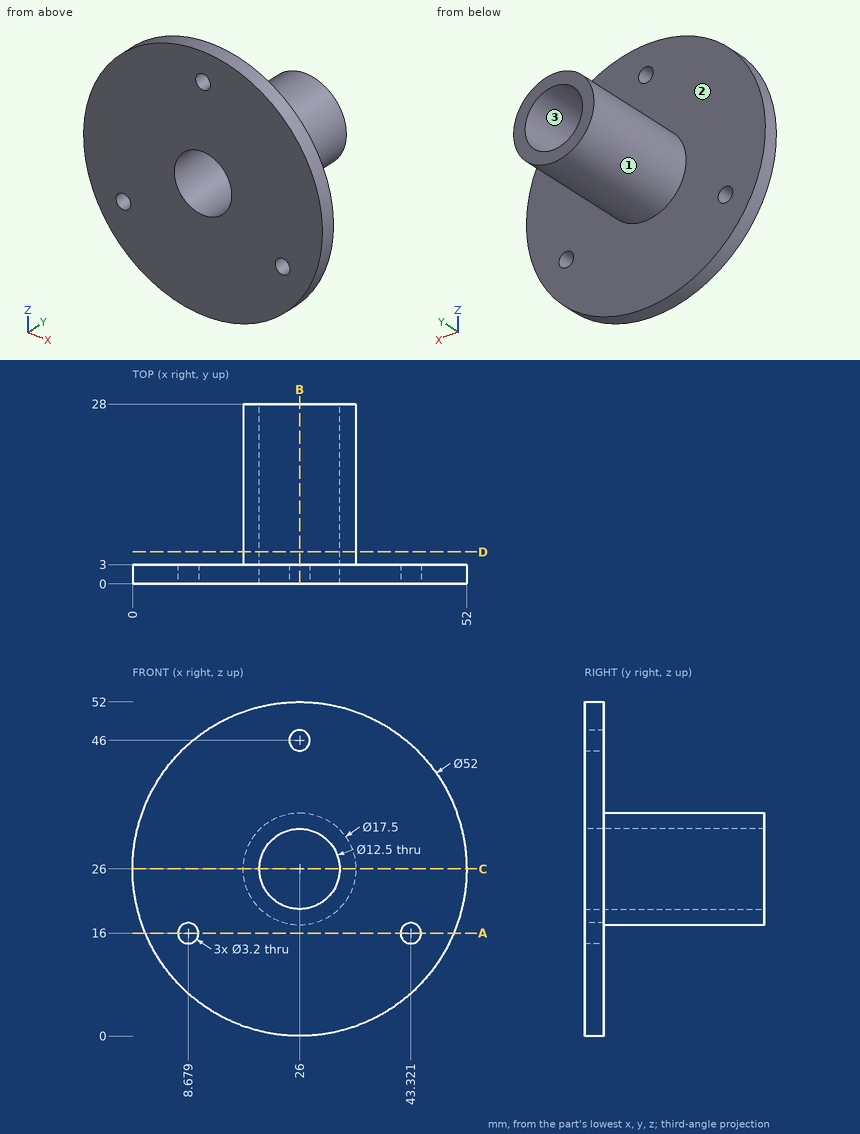
The figure shows three views and two pictorial views of one solid part (mm, origin at its lowest corner). Answer the questions. Coordinates: 2 decimals unless noted, no trailing zeros. Loops run counter-clockwise (first coordinate to the right, second up) from the corner with the lowest first, then second, coordinate; pieces in that order, holes last. Notation, with made-up numbers: M 51,69 L 72,69 A10 ccw 72,84 Z; hole C 53.25,42.25 d8. An arc over 180 degrees is marked long. Answer as CSV lines item,"result". Start each with the question number.
(1) The part is cut by section B-B (x = 26). Give the vertices of the cut face in (y, z).
(2) The part is cut by section A-A (z = 16). Give the vertices of the cut face in (x, y).
(3) The part is cut by section D-D (y = 5). Give the vertices of the cut face in (x, z).
(4) Find the intervals of material crossed by L1, parallel to X at y = 0.75, z = 16; L2, parallel to X at y = 13.5, z = 26; L3, parallel to Y at x = 23.5, z = 14.5, in increasing order. Write a range as [from, to].
(5) Given pin 1 (3 mm diameter, centred on x = 43.32, z = 16, fed in from +Y); pin 2 (4 mm diameter, centred on x = 8.5, z = 12.5, fed in from +Y); pin 3 (12 mm diameter, centred on x = 21, y = 11.5, fed in from -Z); pin 4 (1.5 mm diameter, centred on x = 20.5, y = 16, fed in from -Z), each flat-ended and moving along its own axis, determine where each tip first touches the part or whether it passes through.
(6) The part is cut by section C-C (z = 26). Give the vertices of the cut face in (x, y).
(7) The mould has two halves that part along X. Classify the marked faces 1, 2 and 3: pulls with the +X half, pulls with the -X half, needs draft (parallel to the pull), parting line crosses it, or undercut.
Determined:
1,outline,"M 0,0 L 3,0 L 3,17.25 L 28,17.25 L 28,19.75 L 0,19.75 Z; M 0,32.25 L 28,32.25 L 28,34.75 L 3,34.75 L 3,44.4 L 0,44.4 Z; M 0,47.6 L 3,47.6 L 3,52 L 0,52 Z"
2,outline,"M 2,0 L 7.08,0 L 7.08,3 L 2,3 Z; M 10.28,0 L 41.72,0 L 41.72,3 L 10.28,3 Z; M 44.92,0 L 50,0 L 50,3 L 44.92,3 Z"
3,outline,"C 26,26 d17.5; hole C 26,26 d12.5"
4,L1,"[2, 7.08], [10.28, 41.72], [44.92, 50]"
4,L2,"[17.25, 19.75], [32.25, 34.75]"
4,L3,"[0, 3]"
5,pin 1,"through"
5,pin 2,"y = 3"
5,pin 3,"z = 17.25"
5,pin 4,"z = 18.65"
6,outline,"M 0,0 L 19.75,0 L 19.75,28 L 17.25,28 L 17.25,3 L 0,3 Z; M 32.25,0 L 52,0 L 52,3 L 34.75,3 L 34.75,28 L 32.25,28 Z"
7,face 1,"parting line crosses it"
7,face 2,"needs draft"
7,face 3,"undercut"
